Build history of the part. All positions in model axes, mm. Face numbers are marked on the shaded views. A direction names the side the tool comes from. Round coordinates to 2 decimals unless told otherwise and drop trailing zeros. Write each loop counter-clockwise with the first axis right and the second up, starting at its lowest first coordinate (ties: lowest second). Pieces come first, ordered by that corner, then holes. Notation, with made-up numbers: (82.25, 71.25) -> (95.25, 71.25) arc R29 cw to (95.25, 94.25) -> close; hole circle Ø8 at (-5, 87.5). An arc over 180 degrees is marked (long way). Answer in a Markdown table with one row per item. Add a question column.
from build123d import *

# Parameters (mm, degrees)
CUT_EXTRUDE1_START = -10
CUT_EXTRUDE1_DEPTH = 10
CUT_EXTRUDE2_DEPTH = 2.5
CHAMFER1_SIZE      = 0.8
CHAMFER2_SIZE      = 0.5


with BuildPart() as part:
    # Sketch1 → Revolve1 (revolve)
    with BuildSketch(Plane.XY, mode=Mode.PRIVATE) as revolve1_sk:
        Polygon((-38.5, 0), (-38.5, 4), (-22.5, 4), (-22.5, 5), (0, 5), (0, 6.5), (25.5, 6.5), (25.5, 5), (76, 5), (76, 0), align=None)
    revolve(revolve1_sk.sketch.rotate(Axis((-44.194465138, 0, 0), (1, 0, 0)), 90), axis=Axis((-44.194465138, 0, 0), (1, 0, 0)))

    # Sketch2 → Cut-Extrude1 (cut)
    with BuildSketch(Plane.ZY.offset(38.5).offset(CUT_EXTRUDE1_START)):
        with BuildLine():
            Line((-3.1, -2.527844932), (3.1, -2.527844932))
            ThreePointArc((3.1, -2.527844932), (0, -4), (-3.1, -2.527844932))
        make_face()
        with BuildLine():
            Line((-3.1, 2.527844932), (3.1, 2.527844932))
            ThreePointArc((3.1, 2.527844932), (0, 4), (-3.1, 2.527844932))
        make_face()
    extrude(amount=CUT_EXTRUDE1_DEPTH, mode=Mode.SUBTRACT)

    # Sketch3 → Cut-Extrude2 (cut)
    with BuildSketch(Plane.XY.offset(5)):
        with BuildLine():
            Line((76, -2), (48, -2))
            ThreePointArc((48, -2), (46, 0), (48, 2))
            Line((48, 2), (76, 2))
            ThreePointArc((76, 2), (78, 0), (76, -2))
        make_face()
    extrude(amount=-CUT_EXTRUDE2_DEPTH, mode=Mode.SUBTRACT)

    # Chamfer1
    chamfer1_edges = [part.edges().sort_by_distance(p)[0] for p in [
        (-22.5, 0, -5),
    ]]
    chamfer(chamfer1_edges, length=CHAMFER1_SIZE)

    # Chamfer2
    chamfer2_edges = [part.edges().sort_by_distance(p)[0] for p in [
        (-38.5, -1.341640786, 3.768288736),
        (-38.5, 0, -4),
        (76, 0, -5),
    ]]
    chamfer(chamfer2_edges, length=CHAMFER2_SIZE)


solid = part.part
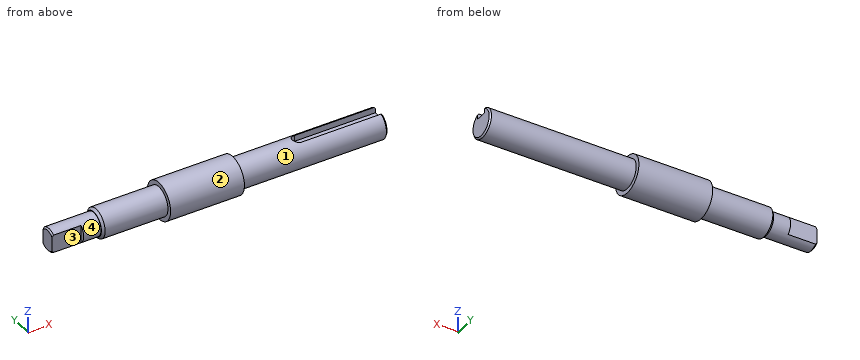
(1) Saw through at D-D (x = 63.5). List the corners of the cut face in (y, z).
(2) Saw through at C-C (x = 5.5). List the corners of the cut face in (y, z).
(3) Saw through at A-A (y = 0). List the corners of the cut face in (x, z).
(4) Probe line 1 along Z through (x, y) = (56, -0.25); line 2 along X through (y, z) = (-3, -1.25); line 3 along X through (y, z) = (5.5, -0.5). List the from-to ranges inside material, lowest first.
(5) Saw through at B-B (z = 0). List the corners of the cut face in (x, y), plus the area to 3 significant figures.
(6) Which spindle directions (+Z, -Z, +X, -X, +Y, -Y) get a long thin tool onto all of the face, cutting with end or side? Do the marked faces 1, 2, 3 and 4. Say none if no direction does.
(7) Drop flat-ended pins along their axis: P1, Ø1.5, axis at x = 1.5, z = -3.5, coming from the +Y side; P2, Ø1.2, axis at y = 3.5, z = 0.5, coming from the -X side; P3, Ø6, axis at x = 24.5, y = -4.5, coming from the +Z side; P4, Ø6, axis at x = 3, y = 3, coming from the -Z side. Give the stop position or say it passes through.
Answer sheet:
| question | item | result |
|---|---|---|
| 1 | outline | (-2, 2.5) -> (-2, 4.58) arc R5 ccw (long way) to (2, 4.58) -> (2, 2.5) -> close |
| 2 | outline | circle Ø13 at (0, 0) |
| 3 | outline | (-38.5, -3.5) -> (-38, -4) -> (-22.5, -4) -> (-22.5, -4.2) -> (-21.7, -5) -> (0, -5) -> (0, -6.5) -> (25.5, -6.5) -> (25.5, -5) -> (75.5, -5) -> (76, -4.5) -> (76, 2.5) -> (46, 2.5) -> (46, 5) -> (25.5, 5) -> (25.5, 6.5) -> (0, 6.5) -> (0, 5) -> (-21.7, 5) -> (-22.5, 4.2) -> (-22.5, 4) -> (-38, 4) -> (-38.5, 3.5) -> close |
| 4 | line 1 | z = -4.99 to 2.5 |
| 4 | line 2 | x = -28.5 to 76 |
| 4 | line 3 | x = 0 to 25.5 |
| 5 | outline | (-38.5, -2.53) -> (-28.5, -2.53) -> (-28.5, -4) -> (-22.5, -4) -> (-22.5, -4.2) -> (-21.7, -5) -> (0, -5) -> (0, -6.5) -> (25.5, -6.5) -> (25.5, -5) -> (75.5, -5) -> (76, -4.5) -> (76, 4.5) -> (75.5, 5) -> (25.5, 5) -> (25.5, 6.5) -> (0, 6.5) -> (0, 5) -> (-21.7, 5) -> (-22.5, 4.2) -> (-22.5, 4) -> (-28.5, 4) -> (-28.5, 2.53) -> (-38.5, 2.53) -> close |
| 5 | area | 1,160 mm² |
| 6 | face 1 | +X |
| 6 | face 2 | +X, -X |
| 6 | face 3 | +Z, -Z, -X, -Y |
| 6 | face 4 | -X |
| 7 | P1 | stops at y = 5.89 |
| 7 | P2 | stops at x = -28.5 |
| 7 | P3 | stops at z = 6.32 |
| 7 | P4 | stops at z = -6.5 |
